from build123d import *

# Parameters (mm, degrees)
F0_R     = 5.7785
F1_DEPTH = 6.35
F2_R     = 6.35


with BuildPart() as f1:
    # F0 (on Top) → F1 (new body)
    with BuildSketch(Plane.XY):
        with BuildLine():
            ThreePointArc((-32.9470856511, 48.2429885797), (-48.9531189835, 48.9531189835), (-48.2429885797, 32.9470856511))
            ThreePointArc((-48.2429885797, 32.9470856511), (-58.42, 0), (-48.2429885797, -32.9470856511))
            ThreePointArc((-48.2429885797, -32.9470856511), (-48.9531189835, -48.9531189835), (-32.9470856511, -48.2429885797))
            ThreePointArc((-32.9470856511, -48.2429885797), (1.5282374195, -58.4000076232), (35.4251532331, -46.4537933695))
            ThreePointArc((35.4251532331, -46.4537933695), (51.8744333617, -46.8373507019), (49.8184745785, -30.5125546401))
            ThreePointArc((49.8184745785, -30.5125546401), (58.4153919217, 0.7337483426), (49.0363490334, 31.7542575646))
            ThreePointArc((49.0363490334, 31.7542575646), (51.7187959431, 48.720604874), (34.622654511, 47.0549486729))
            ThreePointArc((34.622654511, 47.0549486729), (1.0270065512, 58.4109720647), (-32.9470856511, 48.2429885797))
        make_face()
        with Locations((-41.275, -41.275)):
            Circle(F0_R, mode=Mode.SUBTRACT)
        with Locations((43.815, -39.5605)):
            Circle(F0_R, mode=Mode.SUBTRACT)
        with Locations((-41.275, 41.275)):
            Circle(F0_R, mode=Mode.SUBTRACT)
        with Locations((43.815, 41.275)):
            Circle(F0_R, mode=Mode.SUBTRACT)
    extrude(amount=F1_DEPTH)

    # F2
    f2_edges = [f1.edges().sort_by_distance(p)[0] for p in [
        (-48.242989, 32.947086, 3.175),
        (35.425153, -46.453793, 3.175),
        (49.818475, -30.512555, 3.175),
        (-32.947086, 48.242989, 3.175),
        (34.622655, 47.054949, 3.175),
        (49.036349, 31.754258, 3.175),
        (-48.242989, -32.947086, 3.175),
        (-32.947086, -48.242989, 3.175),
    ]]
    fillet(f2_edges, radius=F2_R)


solid = f1.part
Check sheet for the modelled part. Datum: model origin and axes. Units: mm. Round coordinates to 2 decimals unless told otherwise and drop trailing zeros. Write each loop counter-clockwise with the first axis right and the second up, starting at its lowest first coordinate (ties: lowest second). Pieces come first, ordered by that corner, then holes. Notation, with made-up numbers: (-38.5, 88.5) - (-8.5, 88.5) arc R35 cw to (-8.5, 127.5) - close; hole circle Ø10 at (48.25, -38). An arc over 180 degrees is marked (long way). Return JSON: item names as keys, results as strings.
Q1. Cross-section at D-D (y = -23). Record the boundary of the cut face in (x, z), then the cut area to 3 significant figures.
Returned:
{"outline": "(-53.7, 0) - (53.7, 0) - (53.7, 6.35) - (-53.7, 6.35) - close", "area": "682 mm²"}
Q2. Depth check by flat-ended pin: P1, Ø1, axis at x = -32, z = 5, coming from the +Y side; P2, Ø7, axis at x = 43.815, y = 41.275, coming from the +Z side; P3, Ø3, axis at y = -14.5, z = 3, coming from the -X side; P4, Ø1.5, axis at y = 37, z = 3.5, coming from the +X side. Enter the tip coordinate at first touch or a pass-through.
Returned:
{"P1": "stops at y = 49.77", "P2": "passes through", "P3": "stops at x = -56.96", "P4": "stops at x = 54.09"}
Q3. Scan lines: L1, parallel to Y at x = 44, z = 2; L2, parallel to Y at x = -41.5, z = 4.75; L3, parallel to X at y = 36, z = 2. Record each from-to range of solid material in increasing order. Write a range as from..to.
Returned:
{"L1": "y = -50.42..-45.34, -33.78..35.5, 47.05..52.13", "L2": "y = -52.13..-47.05, -35.5..35.5, 47.05..52.13", "L3": "x = -50.77..-43.63, -38.92..41.46, 46.17..53.31"}
Q4. Cross-section at C-C (z = 4). Give the number of separate pieces and of enclosed holes in the cut face, then the cut area to 3 significant figures.
Returned:
{"separate pieces": "1", "enclosed holes": "4", "area": "11,200 mm²"}
Q5. Cross-section at A-A (x = -44.5). Record the boundary of the cut face in (y, z).
Returned:
{"outline": "(-51.64, 0) - (-46.07, 0) - (-46.07, 6.35) - (-51.64, 6.35) - close; (-36.48, 0) - (36.48, 0) - (36.48, 6.35) - (-36.48, 6.35) - close; (46.07, 0) - (51.64, 0) - (51.64, 6.35) - (46.07, 6.35) - close"}
Q6. Draft check along X on faces 1 (the cylindrical face through (58.42, 0.13, 3.13)), 2 (the flat face through (-1, 1, 6.35)), 3 (the cylindrical face through (-35.763, 43.011, 3.131)), 4 (the cylindrical face through (-58.42, 0.43, 3.13)). Enter one of: released by +X, released by -X, zero draft, split by the parting line, or undercut.
Returned:
{"face 1": "released by +X", "face 2": "zero draft", "face 3": "undercut", "face 4": "released by -X"}
Q7. Cross-section at B-B (y = -43.5). Record the boundary of the cut face in (x, z), then the cut area to 3 significant figures.
Returned:
{"outline": "(-51.9, 0) - (-46.61, 0) - (-46.61, 6.35) - (-51.9, 6.35) - close; (-35.94, 0) - (39.59, 0) - (39.59, 6.35) - (-35.94, 6.35) - close; (48.04, 0) - (53.93, 0) - (53.93, 6.35) - (48.04, 6.35) - close", "area": "551 mm²"}
